Autodesk Inventor part; units mm, degrees
ref_plane "YZ Plane" through (0, 0, 0) normal (1, 0, 0) x (0, 1, 0)
ref_plane "XZ Plane" through (0, 0, 0) normal (0, 1, 0) x (-1, 0, 0)
ref_plane "XY Plane" through (0, 0, 0) normal (0, 0, 1) x (1, 0, 0)
sketch "Sketch1" plane through (0, 0, 0) normal (0, 1, 0) x (-1, 0, 0)
  line L0 (0, 0) -> (-50, 0)
  line L1 (-50, -50) -> (0, -50)
  line L2 (-50, -41) -> (-44, -41)
  line L3 (-44, -41) -> (-44, -35)
  line L4 (-44, -35) -> (-50, -35)
  line L5 (-50, -35) -> (-50, -41) construction
  line L6 (-50, -9) -> (-44, -9)
  line L7 (-44, -9) -> (-44, -15)
  line L8 (-44, -15) -> (-50, -15)
  line L9 (-50, -15) -> (-50, -9) construction
  line L10 (-25, 0) -> (-25, -50) construction
  line L11 (-50, -9) -> (-50, 0)
  line L12 (-50, -15) -> (-50, -19)
  line L13 (-50, -41) -> (-50, -50)
  circle A0 centre (-45.75, -5) radius 1.25
  circle A1 centre (-45.75, -45) radius 1.25
  line L14 (-50, -31) -> (-42, -31)
  line L15 (-35, -31) -> (-35, -28.5)
  line L16 (-35, -28.5) -> (-39.7, -28.5)
  line L17 (-50, -19) -> (-42, -19)
  line L18 (-35, -19) -> (-35, -21.5)
  line L19 (-35, -21.5) -> (-39.7, -21.5)
  line L20 (-50, -31) -> (-50, -35)
  line L21 (-50, -28.5) -> (-50, -31) construction
  line L22 (-50, -21.5) -> (-50, -28.5)
  line L23 (-50, -19) -> (-50, -21.5) construction
  line L24 (-42, -32.45) -> (-39.7, -32.45)
  line L25 (-39.7, -32.45) -> (-39.7, -31)
  line L26 (-39.7, -27.05) -> (-42, -27.05)
  line L27 (-42, -27.05) -> (-42, -28.5)
  line L28 (-42, -31) -> (-42, -32.45)
  line L29 (-42, -28.5) -> (-42, -31) construction
  line L30 (-42, -22.95) -> (-39.7, -22.95)
  line L31 (-39.7, -22.95) -> (-39.7, -21.5)
  line L32 (-39.7, -17.55) -> (-42, -17.55)
  line L33 (-42, -17.55) -> (-42, -19)
  line L34 (-42, -21.5) -> (-42, -22.95)
  line L35 (-42, -19) -> (-42, -21.5) construction
  line L36 (-39.7, -28.5) -> (-39.7, -27.05)
  line L37 (-39.7, -31) -> (-39.7, -28.5) construction
  line L38 (-39.7, -21.5) -> (-39.7, -19) construction
  line L39 (-39.7, -19) -> (-39.7, -17.55)
  line L40 (-42, -31) -> (-39.7, -31) construction
  line L41 (-39.7, -31) -> (-35, -31)
  line L42 (-42, -28.5) -> (-50, -28.5)
  line L43 (-39.7, -28.5) -> (-42, -28.5) construction
  line L44 (-42, -21.5) -> (-50, -21.5)
  line L45 (-39.7, -21.5) -> (-42, -21.5) construction
  line L46 (-42, -19) -> (-39.7, -19) construction
  line L47 (-39.7, -19) -> (-35, -19)
  line L48 (0, -41) -> (-6, -41)
  line L49 (-6, -41) -> (-6, -35)
  line L50 (-6, -35) -> (0, -35)
  line L51 (0, -35) -> (0, -41) construction
  line L52 (0, -9) -> (-6, -9)
  line L53 (-6, -9) -> (-6, -15)
  line L54 (-6, -15) -> (0, -15)
  line L55 (0, -15) -> (0, -9) construction
  line L56 (0, -9) -> (0, 0)
  line L57 (0, -15) -> (0, -19)
  line L58 (0, -41) -> (0, -50)
  circle A2 centre (-4.25, -5) radius 1.25
  circle A3 centre (-4.25, -45) radius 1.25
  line L59 (0, -31) -> (-8, -31)
  line L60 (-15, -31) -> (-15, -28.5)
  line L61 (-15, -28.5) -> (-10.3, -28.5)
  line L62 (0, -19) -> (-8, -19)
  line L63 (-15, -19) -> (-15, -21.5)
  line L64 (-15, -21.5) -> (-10.3, -21.5)
  line L65 (0, -31) -> (0, -35)
  line L66 (0, -28.5) -> (0, -31) construction
  line L67 (0, -21.5) -> (0, -28.5)
  line L68 (0, -19) -> (0, -21.5) construction
  line L69 (-8, -32.45) -> (-10.3, -32.45)
  line L70 (-10.3, -32.45) -> (-10.3, -31)
  line L71 (-10.3, -27.05) -> (-8, -27.05)
  line L72 (-8, -27.05) -> (-8, -28.5)
  line L73 (-8, -31) -> (-8, -32.45)
  line L74 (-8, -28.5) -> (-8, -31) construction
  line L75 (-8, -22.95) -> (-10.3, -22.95)
  line L76 (-10.3, -22.95) -> (-10.3, -21.5)
  line L77 (-10.3, -17.55) -> (-8, -17.55)
  line L78 (-8, -17.55) -> (-8, -19)
  line L79 (-8, -21.5) -> (-8, -22.95)
  line L80 (-8, -19) -> (-8, -21.5) construction
  line L81 (-10.3, -28.5) -> (-10.3, -27.05)
  line L82 (-10.3, -31) -> (-10.3, -28.5) construction
  line L83 (-10.3, -21.5) -> (-10.3, -19) construction
  line L84 (-10.3, -19) -> (-10.3, -17.55)
  line L85 (-8, -31) -> (-10.3, -31) construction
  line L86 (-10.3, -31) -> (-15, -31)
  line L87 (-8, -28.5) -> (0, -28.5)
  line L88 (-10.3, -28.5) -> (-8, -28.5) construction
  line L89 (-8, -21.5) -> (0, -21.5)
  line L90 (-10.3, -21.5) -> (-8, -21.5) construction
  line L91 (-8, -19) -> (-10.3, -19) construction
  line L92 (-10.3, -19) -> (-15, -19)
  dimension "d0" = 50
  dimension "d1" = 50
  dimension "d20" = 6
  dimension "d21" = 6
  dimension "d22" = 6
  dimension "d26" = 20
  dimension "d27" = 2.5
  dimension "d28" = 4.25
  dimension "d30" = 2.5
  dimension "d31" = 4.25
  dimension "d32" = 4
  dimension "d33" = 15
  dimension "d34" = 2.5
  dimension "d35" = 15
  dimension "d36" = 2.5
  dimension "d37" = 4
  dimension "d38" = 5.4
  dimension "d39" = 2.3
  dimension "d40" = 8
  dimension "d41" = 2.3
  dimension "d42" = 5.4
  dimension "d43" = 8
  dimension "d44" = 4
extrude "Extrusion2" add sketch "Sketch1" along normal blind 6
equation "\"d22\" = d21"
equation "\"d30\" = d27"
equation "\"d31\" = d28"
equation "\"d32\" = d44"
equation "\"d33\" = d35"
equation "\"d34\" = d27"
equation "\"d36\" = d27"
equation "\"d43\" = d40"
properties part number "wall-front"
Geometry: final body of the model. Coordinates: model frame, mm. A direction names the side the tool comes from. Give positions to 0.01 mm unless a question says otherwise; leave off trailing zeros. Order: outer loops, then holes, each group sorted by start corner. A loop starts at its lowest first (then second) coordinate and runs counter-clockwise, first axis right, second up. Notation, with made-up numbers: (53.25, -18) - (94.25, -18) arc R17 ccw to (94.25, 7) - close; hole circle Ø3 at (-5, 74). An arc over 180 degrees is marked (long way). Use CSV: the item, a comma, the result in double quotes.
1. Section query C-C (z = -5). Output: boundary loops of the cut face in (x, y), plus the area to 3 significant figures.
Answers below:
outline,"(0, 0) - (3, 0) - (3, 6) - (0, 6) - close; (5.5, 0) - (44.5, 0) - (44.5, 6) - (5.5, 6) - close; (47, 0) - (50, 0) - (50, 6) - (47, 6) - close"
area,"270 mm2"
2. Section query D-D (y = 4.7). Give the number of separate pieces and of enclosed holes in the cut face, plus the area to 3 significant figures.
Answers below:
separate pieces,"1"
enclosed holes,"4"
area,"2,160 mm2"
3. Section query B-B (x = 4.25). Output: boundary loops of the cut face in (y, z).
Answers below:
outline,"(0, -50) - (6, -50) - (6, -46.25) - (0, -46.25) - close; (0, -43.75) - (6, -43.75) - (6, -41) - (0, -41) - close; (0, -35) - (6, -35) - (6, -31) - (0, -31) - close; (0, -28.5) - (6, -28.5) - (6, -21.5) - (0, -21.5) - close; (0, -19) - (6, -19) - (6, -15) - (0, -15) - close; (0, -9) - (6, -9) - (6, -6.25) - (0, -6.25) - close; (0, -3.75) - (6, -3.75) - (6, 0) - (0, 0) - close"
4. Mould query, pull axis X, two halves, no side actions, for faces 4 (the face through (8, 3, -22)), 5 (the face through (37, 3, -19)), 6 (the face through (0, 3, -33)). Classes: +X half, -X half, draft (parallel to the pull), parting line (faces both ways), or undercut.
Answers below:
face 4,"undercut"
face 5,"draft"
face 6,"-X half"
5. Access query for faces 1 (the face through (4, 3, -31)), 2 (the face through (9, 3, -27.05)), 3 (the face through (35, 3, -20)). Directions: +Z, -Z, +X, -X, +Y, -Y. A direction counts if a zero-diameter tool reaches every point of the face in a straight line with its end or side. Return the directions, or none.
Answers below:
face 1,"-X, +Y, -Y"
face 2,"+Y, -Y"
face 3,"+X, +Y, -Y"
6. Material intervals for line 1 along Z through (x, y) = (9, 2.3); line 2 along Z through (x, y) = (13.5, 5.6); line 3 along X through (y, z) = (3.9, -4), sorted ascending. Write a range as from..to.
Answers below:
line 1,"-50..-32.45, -27.05..-22.95, -17.55..0"
line 2,"-50..-31, -28.5..-21.5, -19..0"
line 3,"0..3.5, 5..45, 46.5..50"
7. Contact query for a flat-ended pin moving along its axis: pin 1 (1.8 mm diameter, centred on y = 4.5, z = -10.5, fed in from +X). Output: stop coordinate, or through.
Answers below:
pin 1,"x = 44"
8. Section query A-A (x = 36). Output: boundary loops of the cut face in (y, z).
Answers below:
outline,"(0, -50) - (6, -50) - (6, -31) - (0, -31) - close; (0, -28.5) - (6, -28.5) - (6, -21.5) - (0, -21.5) - close; (0, -19) - (6, -19) - (6, 0) - (0, 0) - close"
